The model under review builds one solid part; all positions refer to its coordinate system, in mm. A direction names the side the tool comes from. Coordinates: 2 decimals unless noted, no trailing zeros. Write each loop counter-clockwise with the first axis right and the second up, starting at its lowest first coordinate (ties: lowest second). Pieces come first, ordered by that corner, then holes. Notation, with made-up numbers: (5, 3.5) - (17, 3.5) arc R11 cw to (17, 7.5) - close; hole circle Ø1 at (-22.75, 73.25). An arc over 180 degrees is marked (long way). Put each result on its own line as item: value. Start each with the question number.
Item 1: Consider section C-C on y = 62.5. Give the boundary of the cut face in (x, z), then the cut area to 3 significant figures.
Item 2: For pin 1 (17 mm diameter, centred on y = 30, z = 42.5, fed in from -X); pin 2 (2 mm diameter, centred on x = 54.5, y = 65, fed in from +Z), all flat-tipped, find the tip position at first contact; note any pin that passes through.
Item 3: To check wall thickness, follow L1, parallel to Y at x = 54.5, z = 44; L2, parallel to X at y = 73, z = 36; L3, parallel to Y at x = 36, z = 25. State the ranges of each line that lie inside material, in increasing order. Write a range as [from, to].
Item 4: Consider section A-A on x = 36. Give the boundary of the cut face in (y, z).
Item 5: Consider section D-D on x = 93.5. Give the boundary of the cut face in (y, z), then the cut area to 3 significant figures.
Item 6: Machinability: for faces 4 (the face through (96.5, 39, 31)), 5 (the face through (35, 1, 35)), 6 (the face through (49, 80, 30)), which of the approach directions +Z, -Z, +X, -X, +Y, -Y give a long, thin tool a straight path to every point of the face, cutting with its end or side? Answer none if there is none.
Item 7: Consider section B-B on z = 37.5. Give the boundary of the cut face in (x, y).
Item 8: Mouldability with a two-part tool opening along Z and no side actions: class faces 1 (the face through (0, 39, 30)), 2 (the face through (25, 1, 29)), 3 (the face through (46, 2, 60)) as pulls with the +Z half, pulls with the -Z half, needs draft (parallel to the pull), parting line crosses it, or undercut.
```python
from build123d import *

# Parameters (mm, degrees)
ESBO_O1_W                  = 100
ESBO_O1_H                  = 80
RESSALTO_EXTRUS_O1_DEPTH   = 3
ESBO_O2_W                  = 100
ESBO_O2_H                  = 80
ESBO_O2_W_2                = 93
ESBO_O2_H_2                = 74.4
RESSALTO_EXTRUS_O2_DEPTH   = 60
ESBO_O3_W                  = 19.7
ESBO_O3_H                  = 13
CORTE_EXTRUS_O1_DEPTH      = 10
CORTE_EXTRUS_O1_DEPTH_BACK = 17


with BuildPart() as part:
    # Esboço1 → Ressalto-extrusão1 (new body)
    with BuildSketch(Plane.XY):
        with Locations((50, 40)):
            Rectangle(ESBO_O1_W, ESBO_O1_H)
    extrude(amount=RESSALTO_EXTRUS_O1_DEPTH)

    # Esboço2 → Ressalto-extrusão2 (add)
    with BuildSketch(Plane.XY):
        with Locations((50, 40)):
            Rectangle(ESBO_O2_W, ESBO_O2_H)
        with Locations((50, 40)):
            Rectangle(ESBO_O2_W_2, ESBO_O2_H_2, mode=Mode.SUBTRACT)
    extrude(amount=RESSALTO_EXTRUS_O2_DEPTH)

    # Esboço3 → Corte-extrusão1 (cut, two sides)
    with BuildSketch(Plane(origin=(0, 0, 0), x_dir=(1, 0, 0), z_dir=(0, 1, 0))) as corte_extrus_o1_sk:
        with Locations((34.85, -28.5)):
            Rectangle(ESBO_O3_W, ESBO_O3_H)
    extrude(amount=CORTE_EXTRUS_O1_DEPTH, mode=Mode.SUBTRACT)
    extrude(corte_extrus_o1_sk.sketch, amount=-CORTE_EXTRUS_O1_DEPTH_BACK, mode=Mode.SUBTRACT)


solid = part.part
```
Report:
1. outline: (0, 0) - (100, 0) - (100, 60) - (96.5, 60) - (96.5, 3) - (3.5, 3) - (3.5, 60) - (0, 60) - close
1. area: 699 mm²
2. pin 1: x = 0
2. pin 2: z = 3
3. L1: [0, 2.8], [77.2, 80]
3. L2: [0, 3.5], [96.5, 100]
3. L3: [77.2, 80]
4. outline: (0, 0) - (80, 0) - (80, 60) - (77.2, 60) - (77.2, 3) - (2.8, 3) - (2.8, 22) - (0, 22) - close; (0, 35) - (2.8, 35) - (2.8, 60) - (0, 60) - close
5. outline: (0, 0) - (80, 0) - (80, 60) - (77.2, 60) - (77.2, 3) - (2.8, 3) - (2.8, 60) - (0, 60) - close
5. area: 559 mm²
6. face 4: +Z
6. face 5: -Y
6. face 6: +Z, -Z, +X, -X, +Y
7. outline: (0, 0) - (100, 0) - (100, 80) - (0, 80) - close; hole (3.5, 2.8) - (96.5, 2.8) - (96.5, 77.2) - (3.5, 77.2) - close
8. face 1: needs draft
8. face 2: undercut
8. face 3: pulls with the +Z half
